Drawing for the job (mm, zero at the part's lowest x, y, z). Coordinates: 2 decimals unless noted, no trailing zeros. Write each loop counter-clockwise with the first axis right and the second up, starting at its lowest first coordinate (ties: lowest second). Pieces come first, ordered by that corner, then holes. Notation, with made-up numbers: M -18,-6 L 34,-6 A23 ccw 34,29 Z; hole C 21,-22.5 d6. An arc over 180 degrees is marked long. Use CSV: the item, a comma, the result in double quotes. Start each with the question number.
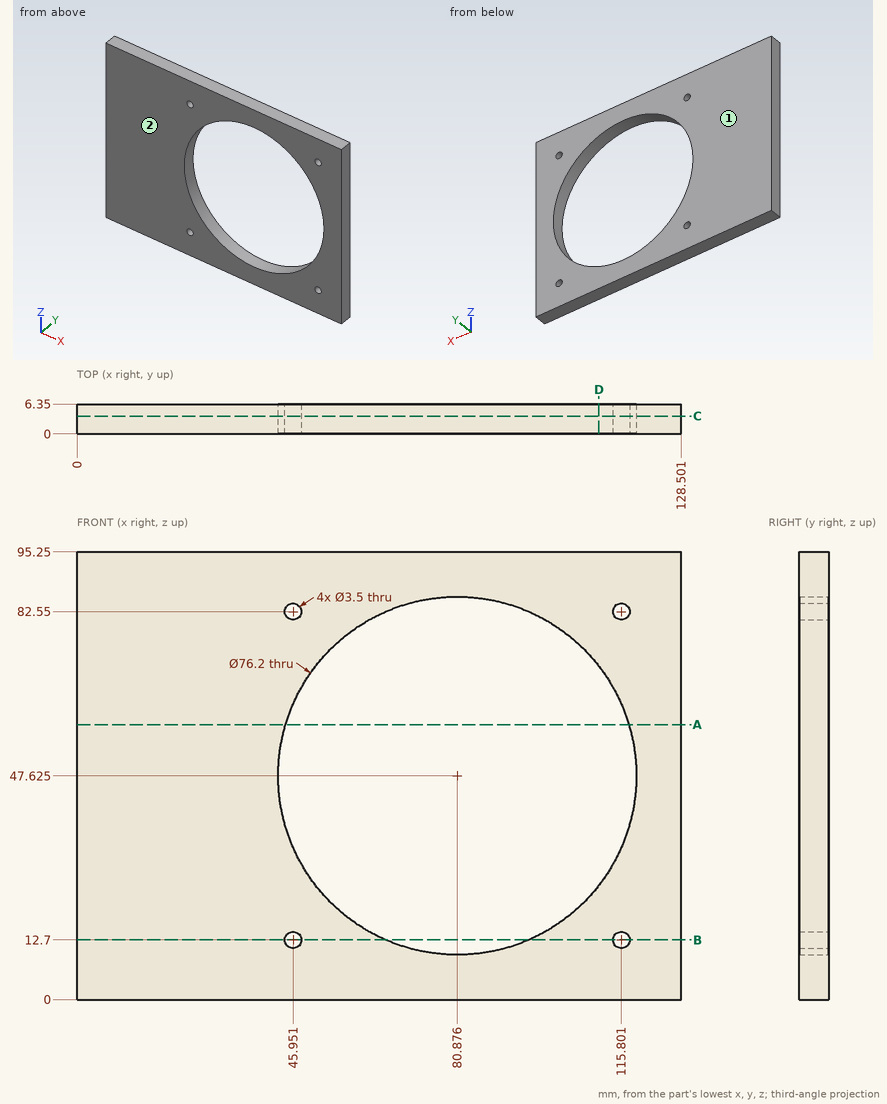
1) Drop a flat-ended pin along its axis: P1, Ø5.5, axis at x = 115.8, z = 82.55, coming from the +Y side. Give the stop position or say it passes through.
2) Wall check: L1, parallel to Z at x = 54, y = 0.5; L2, parallel to Z at x = 98, y = 4.5; L3, parallel to X at y = 4.5, z = 44.5 (1 decimal). Give the ranges that are in metal, low to high. Write a range as [from, to].
3) Band-saw the part on B-B on z = 12.7. List the corners of the cut face in (x, y), then the cut area to 3 significant figures.
4) Band-saw the part on A-A on z = 58.5. List the corners of the cut face in (x, y), then the cut area to 3 significant figures.
5) Band-saw the part on C-C on y = 3.75. State how many separate pieces and enclosed holes the cut face has, then the cut area to 3 significant figures.
6) Two-plate mould, pull along Y, no slides. Class the marked faces 1 and 2: pulls with the +Y half, pulls with the -Y half, needs draft (parallel to the pull), parting line crosses it, or undercut.
7) Band-saw the part on D-D on x = 111. List the corners of the cut face in (y, z).
Findings below:
1,P1,"stops at y = 6.35"
2,L1,"z = [0, 20.62], [74.63, 95.25]"
2,L2,"z = [0, 13.59], [81.66, 95.25]"
2,L3,"x = [0, 42.9], [118.8, 128.5]"
3,outline,"M 0,0 L 44.2,0 L 44.2,6.35 L 0,6.35 Z; M 47.7,0 L 65.65,0 L 65.65,6.35 L 47.7,6.35 Z; M 96.1,0 L 114.05,0 L 114.05,6.35 L 96.1,6.35 Z; M 117.55,0 L 128.5,0 L 128.5,6.35 L 117.55,6.35 Z"
3,area,"578 mm2"
4,outline,"M 0,0 L 44.36,0 L 44.36,6.35 L 0,6.35 Z; M 117.39,0 L 128.5,0 L 128.5,6.35 L 117.39,6.35 Z"
4,area,"352 mm2"
5,separate pieces,"1"
5,enclosed holes,"5"
5,area,"7,640 mm2"
6,face 1,"pulls with the +Y half"
6,face 2,"pulls with the -Y half"
7,outline,"M 0,0 L 6.35,0 L 6.35,24.3 L 0,24.3 Z; M 0,70.95 L 6.35,70.95 L 6.35,95.25 L 0,95.25 Z"
